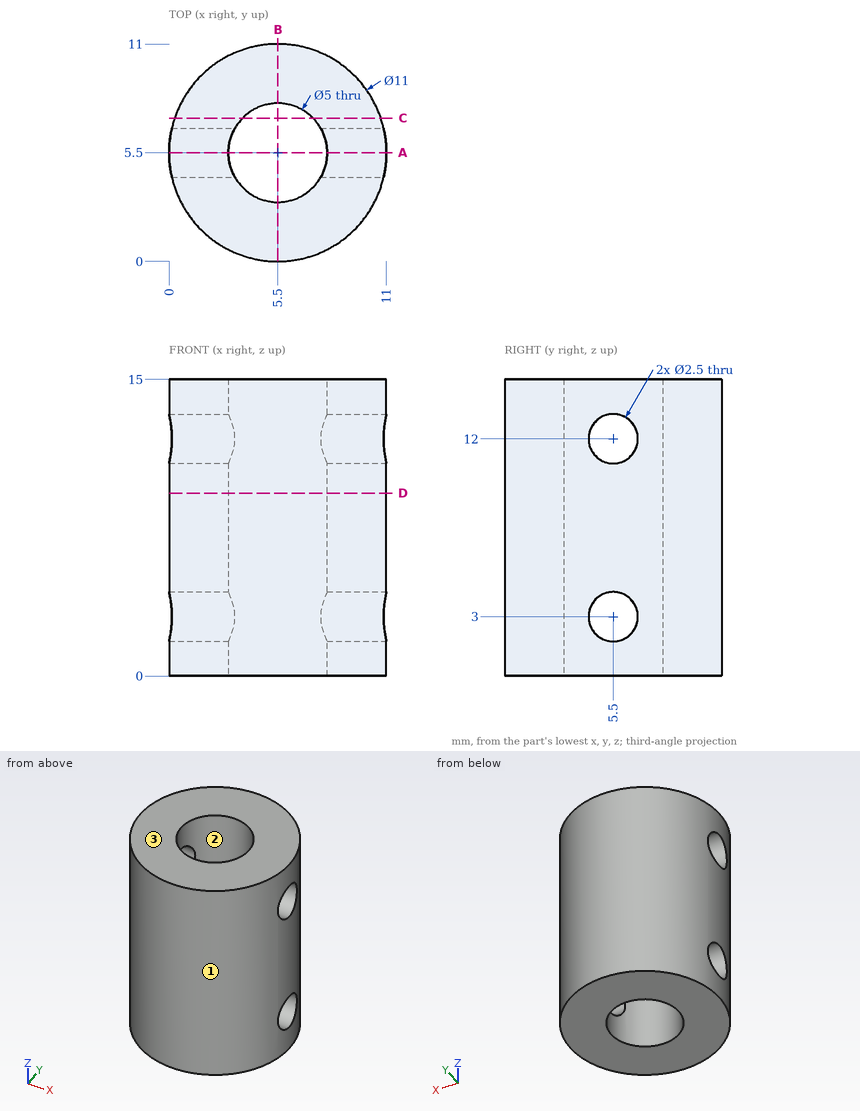
The figure shows three views and two pictorial views of one solid part (mm, origin at its lowest corner). Answer the questions. Coordinates: 2 decimals unless noted, no trailing zeros. Write each loop counter-clockwise with the first axis right and the second up, starting at its lowest first coordinate (ties: lowest second). Pieces come first, ordered by that corner, then holes. Notation, with made-up numbers: (-2.5, -14.5) -> (44.5, -14.5) arc R32 cw to (44.5, 23.5) -> close; hole circle Ø11 at (6, -13). An arc over 180 degrees is marked (long way). Return JSON: item names as keys, results as strings.
1. A cutting plane is placed at B-B (x = 5.5). Determine the outline of the cut face in (y, z).
Found:
{"outline": "(0, 0) -> (3, 0) -> (3, 15) -> (0, 15) -> close; (8, 0) -> (11, 0) -> (11, 15) -> (8, 15) -> close"}
2. Find the intervals of material crossed by line 1 along Y through (x, z) = (5.5, 7.75); line 2 along Y through (x, z) = (8.85, 12); line 3 along X through (y, z) = (4.75, 6), in increasing order. Write a range as from..to.
Found:
{"line 1": "0..3, 8..11", "line 2": "1.14..4.25, 6.75..9.86", "line 3": "0.05..3.12, 7.88..10.95"}
3. Determine the mould class of the marked faces 1, 2 and 3 for opening direction X: pulls with the +X half, pulls with the -X half, needs draft (parallel to the pull), parting line crosses it, or undercut.
Found:
{"face 1": "parting line crosses it", "face 2": "undercut", "face 3": "needs draft"}
4. A cutting plane is placed at C-C (y = 7.25). Determine the outline of the cut face in (x, z).
Found:
{"outline": "(0.29, 0) -> (3.71, 0) -> (3.71, 15) -> (0.29, 15) -> close; (7.29, 0) -> (10.71, 0) -> (10.71, 15) -> (7.29, 15) -> close"}
5. A cutting plane is placed at A-A (y = 5.5). Determine the outline of the cut face in (x, z).
Found:
{"outline": "(0, 0) -> (3, 0) -> (3, 1.75) -> (0, 1.75) -> close; (0, 4.25) -> (3, 4.25) -> (3, 10.75) -> (0, 10.75) -> close; (0, 13.25) -> (3, 13.25) -> (3, 15) -> (0, 15) -> close; (8, 0) -> (11, 0) -> (11, 1.75) -> (8, 1.75) -> close; (8, 4.25) -> (11, 4.25) -> (11, 10.75) -> (8, 10.75) -> close; (8, 13.25) -> (11, 13.25) -> (11, 15) -> (8, 15) -> close"}
6. A cutting plane is placed at D-D (z = 9.25). Determine the outline of the cut face in (x, y), and give its area (3 significant figures).
Found:
{"outline": "circle Ø11 at (5.5, 5.5); hole circle Ø5 at (5.5, 5.5)", "area": "75.4 mm2"}
7. Each of these flat-tipped pins is pushed along its axis until it touches: P1, Ø5, axis at x = 9, z = 7.5, coming from the -Y side; P2, Ø2, axis at y = 4, z = 13.5, coming from the +X side; P3, Ø5, axis at y = 10, z = 3, coming from the -X side. Where does it stop, or does it pass through?
Found:
{"P1": "y = 0.09", "P2": "x = 10.98", "P3": "x = 0.38"}
